Here's how the part is built. I have some questions about the finished solid (model axes, mm). A direction names the side the tool comes from. Coordinates: 2 decimals unless noted, no trailing zeros. Loops run counter-clockwise (first coordinate to the right, second up) from the corner with the lowest first, then second, coordinate; pieces in that order, holes last. Notation, with made-up numbers: M 67.5,46 L 104.5,46 A27 cw 104.5,65 Z; hole C 65.5,66 d11. An arc over 180 degrees is marked long. Use one line per item in the form item = value. Start each with the question number.
(1) Imagine slicing it at D-D, the plane x = 35. Please give me the cut outline in (y, z) (1 decimal).
(2) Please list where these lines run through material, in increasing order: L1, parallel to Z at x = 0, y = -4.9; L2, parallel to Z at x = 0, y = 3.5; L3, parallel to Z at x = 43, y = 0.75.
(3) Imagine slicing it at C-C, the plane x = 3.5. Please give me the cut outline in (y, z) (1 decimal), and give its area (3 significant figures).
(4) Thinking about a two-plate mould opening in Z: for faces 4 (the flat face through (25, 0, 25.4)), 5 (the cylindrical face through (41.408, -1.986, 18.465)), 6 (the flat face through (21, -7.938, 0)), 7 (the flat face through (1.4, -3.175, 18.2)), which applies, +Z half, -Z half, draft (parallel to the pull), parting line (faces both ways), or undercut?
(5) Imagine slicing it at A-A, the plane z = 9.5. Please give me the cut outline in (x, y) (1 decimal).
(6) Will these pins go through, and if not, where does the flat tip stop? P1, Ø8.5, axis at y = 0, z = -15.875, coming from the -X side; P2, Ø7.5, axis at y = 0, z = 15.875, coming from the -X side; P3, Ø4, axis at y = 2, z = -17.5, coming from the -X side.
(7) On a 3-axis mill with a long thin cutter (end or side, diameter ignored), from which of +Z, -Z, +X, -X, +Y, -Y can I reach the whole of each face in a straight line? I mean faces 1 (the cylindrical face through (-25.394, 0.111, -0.559)), 2 (the cylindrical face through (-2.682, 2.459, -20.424)), 3 (the flat face through (31.75, 0, 16)). Say none if no direction works.
(8) Imagine slicing it at B-B, the plane y = 6.5. Please give me the cut outline in (x, z).
```python
from build123d import *

# Parameters (mm, degrees)
SKETCH1_W           = 76.2
SKETCH1_H           = 50.8
BOSS_EXTRUDE1_DEPTH = 7.9375
SKETCH2_R           = 20.5994
CUT_EXTRUDE1_DEPTH  = 11.1125
SKETCH3_R           = 18.0975
CUT_EXTRUDE2_DEPTH  = 12.7
SKETCH7_R           = 3.2639
CUT_EXTRUDE6_DEPTH  = 19.05
CUT_EXTRUDE7_DEPTH  = 16.875


with BuildPart() as part:
    # Sketch1 → Boss-Extrude1 (new body, symmetric)
    with BuildSketch(Plane(origin=(0, 0, 0), x_dir=(1, 0, 0), z_dir=(0, 1, 0))):
        with Locations((12.7, 0)):
            Rectangle(SKETCH1_W, SKETCH1_H)
    extrude(amount=BOSS_EXTRUDE1_DEPTH, both=True)

    # Sketch2 → Cut-Extrude1 (cut)
    with BuildSketch(Plane(origin=(0, 7.9375, 0), x_dir=(1, 0, 0), z_dir=(0, 1, 0))):
        Circle(SKETCH2_R)
    extrude(amount=-CUT_EXTRUDE1_DEPTH, mode=Mode.SUBTRACT)

    # Sketch3 → Cut-Extrude2 (cut)
    with BuildSketch(Plane(origin=(0, -3.175, 0), x_dir=(1, 0, 0), z_dir=(0, 1, 0))):
        Circle(SKETCH3_R)
    extrude(amount=-CUT_EXTRUDE2_DEPTH, mode=Mode.SUBTRACT)

    # Sketch7 → Cut-Extrude6 (cut)
    with BuildSketch(Plane(origin=(50.8, 0, 0), x_dir=(0, 0, -1), z_dir=(1, 0, 0))):
        with Locations((-15.875, 0)):
            Circle(SKETCH7_R)
        with Locations((15.875, 0)):
            Circle(SKETCH7_R)
    extrude(amount=-CUT_EXTRUDE6_DEPTH, mode=Mode.SUBTRACT)

    # Sketch8 → Cut-Extrude7 (cut, through all)
    with BuildSketch(Plane(origin=(0, 7.9375, 0), x_dir=(1, 0, 0), z_dir=(0, 1, 0))):
        with BuildLine():
            Line((0, -25.4), (0, -38.1))
            Line((0, -38.1), (-50.8, -38.1))
            Line((-50.8, -38.1), (-50.8, 38.1))
            Line((-50.8, 38.1), (0, 38.1))
            Line((0, 38.1), (0, 25.4))
            ThreePointArc((0, 25.4), (-25.4, 0), (0, -25.4))
        make_face()
    extrude(amount=-CUT_EXTRUDE7_DEPTH, mode=Mode.SUBTRACT)


solid = part.part
```
Answer:
q1.outline = M -7.9,-25.4 L 7.9,-25.4 L 7.9,25.4 L -7.9,25.4 Z; hole C 0,-15.9 d6.5; hole C 0,15.9 d6.5
q2.L1 = -25.4 to -18.1, 18.1 to 25.4
q2.L2 = -25.4 to -20.6, 20.6 to 25.4
q2.L3 = -25.4 to -19.05, -12.7 to 12.7, 19.05 to 25.4
q3.outline = M -7.9,-25.4 L 7.9,-25.4 L 7.9,-20.3 L -3.2,-20.3 L -3.2,-17.8 L -7.9,-17.8 Z; M -7.9,17.8 L -3.2,17.8 L -3.2,20.3 L 7.9,20.3 L 7.9,25.4 L -7.9,25.4 Z
q3.area = 186 mm²
q4.face_4 = +Z half
q4.face_5 = undercut
q4.face_6 = draft
q4.face_7 = undercut
q5.outline = M -23.6,-7.9 L -15.4,-7.9 L -15.4,-3.2 L -18.3,-3.2 L -18.3,7.9 L -23.6,7.9 Z; M 15.4,-7.9 L 50.8,-7.9 L 50.8,7.9 L 18.3,7.9 L 18.3,-3.2 L 15.4,-3.2 Z
q6.P1 = -22.58
q6.P2 = -22.32
q6.P3 = -20.12
q7.face_1 = -X, +Y, -Y
q7.face_2 = +Y
q7.face_3 = +X
q8.outline = M 0,-25.4 L 50.8,-25.4 L 50.8,25.4 L 0,25.4 A25.4 ccw Z; hole C 0,0 d41.2
